The listing builds one solid part. Answer for the finished solid, in the listing's coordinates (mm). Face numbers are marked on the shaded views. Round coordinates to 2 decimals unless told otherwise and drop trailing zeros. Order: outer loops, then holes, each group sorted by start corner. A loop starts at its lowest first (then second) coordinate and runs counter-clockwise, first axis right, second up. Notation, with made-up numbers: M 24,81.25 L 43,81.25 A12 ccw 43,91.25 Z; hole C -30,68.5 d6. An arc over 180 degrees is marked long. Write item = value, one per line. Start each with the question number.
(1) A cutting plane is placed at B-B, the plane x = 230.5. Determine the outline of the cut face in (y, z) (3 decimals).
(2) Each of these flat-tipped pins is pushed along its axis until it touches: pin 1 (1.6 mm diameter, centred on y = 14, z = 23, fed in from -X); pin 2 (2.5 mm diameter, centred on y = 14.5, z = 23.5, fed in from +X). Where does it stop, or does it pass through?
(3) A cutting plane is placed at A-A, the plane y = 14. Determine the outline of the cut face in (x, z) (3 decimals), and give its area (3 significant figures).
(4) A cutting plane is placed at C-C, the plane x = 379.74. Determine the outline of the cut face in (y, z) (3 decimals).
(5) Straight lines are drawn through the part: probe 1 along Y at (x, z) = (350.5, 4.5) (3 decimals); probe 2 along X at (y, z) = (15, 22.5). For each, find the intervals that lie inside material, in ascending order. Write a range as from..to.
(6) For a pull along Y with two mould halves and no side action, classify the marked faces 1, 2 and 3 as released by +Y, released by -Y, zero draft, split by the parting line, or undercut.
from build123d import *

# Parameters (mm, degrees)
SKETCH1_W           = 395.5
SKETCH1_H           = 25.4
SKETCH1_R           = 3.175
BOSS_EXTRUDE1_DEPTH = 25.4
CUT_EXTRUDE1_REACH  = 399.128
SKETCH2_W           = 19.05
SKETCH2_H           = 19.05
SKETCH4_W           = 25.4
SKETCH4_H           = 19.05
CUT_EXTRUDE2_DEPTH  = 38.1
FILLET1_R           = 20


with BuildPart() as part:
    # Sketch1 → Boss-Extrude1 (new body)
    with BuildSketch(Plane(origin=(0, 0, 0), x_dir=(1, 0, 0), z_dir=(0, 1, 0))):
        with Locations((197.75, -12.7)):
            Rectangle(SKETCH1_W, SKETCH1_H)
        with Locations(Location((197.75, -12.7, 0), (0, 0, 270))):
            Circle(SKETCH1_R, mode=Mode.SUBTRACT)
        with Locations(Location((15.76, -12.7, 0), (0, 0, 270))):
            Circle(SKETCH1_R, mode=Mode.SUBTRACT)
        with Locations(Location((379.74, -12.7, 0), (0, 0, 90))):
            Circle(SKETCH1_R, mode=Mode.SUBTRACT)
    extrude(amount=BOSS_EXTRUDE1_DEPTH)

    # Cut-Extrude1: up to this face of the body (flat: up to its plane)
    cut_extrude1_end = Plane(part.part.faces().sort_by_distance((395.5, 12.7, 12.7))[0])
    # Sketch2 → Cut-Extrude1 (cut, up to the picked face)
    with BuildSketch(Plane.ZY, mode=Mode.PRIVATE) as cut_extrude1_sk1:
        with Locations((12.7, 12.7)):
            Rectangle(SKETCH2_W, SKETCH2_H)
    cut_extrude1_tool1 = split(extrude(cut_extrude1_sk1.sketch, amount=-CUT_EXTRUDE1_REACH, mode=Mode.PRIVATE), bisect_by=cut_extrude1_end, keep=Keep.BOTH, mode=Mode.PRIVATE)
    add(cut_extrude1_tool1.solids().sort_by(Axis((0, 12.7, 12.7), (1, 0, 0)))[0], mode=Mode.SUBTRACT)

    # Sketch4 → Cut-Extrude2 (cut)
    with BuildSketch(Plane.ZY):
        with Locations((12.7, 12.7)):
            Rectangle(SKETCH4_W, SKETCH4_H)
    cut_extrude2 = extrude(amount=-CUT_EXTRUDE2_DEPTH, mode=Mode.SUBTRACT)

    # Mirror1: Cut-Extrude2 across plane
    add(cut_extrude2.mirror(Plane.ZY.offset(-197.75)), mode=Mode.SUBTRACT)

    # Fillet1
    # the kernel refuses this fillet: 20 mm, written as the material it takes off along each edge
    with BuildSketch(Plane(origin=(395.5, -50, 0), x_dir=(-1, 0, 0), z_dir=(0, 1, 0)), Plane(origin=(395.5, -27.775, 0), x_dir=(-1, 0, 0), z_dir=(0, 1, 0)), Plane(origin=(0, -27.775, 25.4), x_dir=(1, 0, 0), z_dir=(0, 1, 0))) as fillet1_piece_1:
        with BuildLine():
            CenterArc((FILLET1_R, FILLET1_R), FILLET1_R, 180, 90)
            Line((0, FILLET1_R), (0, 0))
            Line((0, 0), (FILLET1_R, 0))
        make_face()
    extrude(amount=103.175, mode=Mode.SUBTRACT)
    with BuildSketch(Plane(origin=(395.5, -50, 25.4), x_dir=(-1, 0, 0), z_dir=(0, 1, 0)), Plane(origin=(395.5, -27.775, 25.4), x_dir=(-1, 0, 0), z_dir=(0, 1, 0)), Plane(origin=(0, -50, 25.4), x_dir=(0, 0, -1), z_dir=(0, 1, 0)), Plane(origin=(0, -50, 0), x_dir=(1, 0, 0), z_dir=(0, 1, 0)), Plane(origin=(0, -27.775, 0), x_dir=(1, 0, 0), z_dir=(0, 1, 0))) as fillet1_piece_2:
        with BuildLine():
            CenterArc((FILLET1_R, -FILLET1_R), FILLET1_R, 90, 90)
            Line((0, -FILLET1_R), (0, 0))
            Line((0, 0), (FILLET1_R, 0))
        make_face()
    extrude(amount=103.175, mode=Mode.SUBTRACT)


solid = part.part
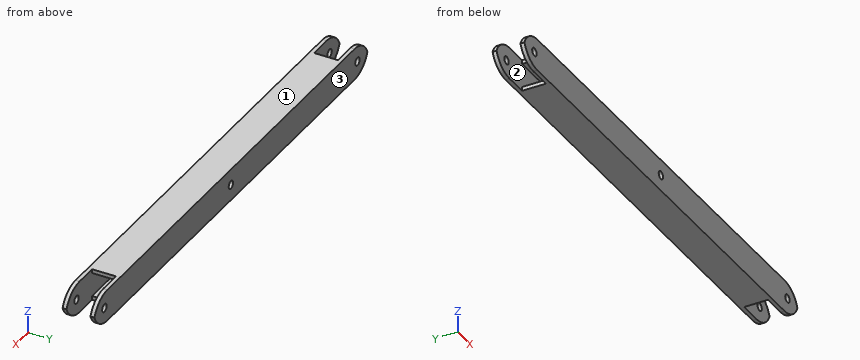
Reported:
q1.outline = M 0,0 L 25.4,0 L 25.4,25.4 L 0,25.4 Z; hole M 3.175,3.175 L 22.225,3.175 L 22.225,22.225 L 3.175,22.225 Z
q2.pin_1 = 38.1
q2.pin_2 = 357.4
q3.outline = M 38.1,0 L 357.4,0 L 357.4,3.175 L 38.1,3.175 Z; M 38.1,22.225 L 357.4,22.225 L 357.4,25.4 L 38.1,25.4 Z
q3.area = 2,030 mm²
q4.outline = M 0,0.455 L 3.175,0.455 L 3.175,9.525 L 0,9.525 Z; M 0,15.875 L 3.175,15.875 L 3.175,24.945 L 0,24.945 Z; M 22.225,0.455 L 25.4,0.455 L 25.4,9.525 L 22.225,9.525 Z; M 22.225,15.875 L 25.4,15.875 L 25.4,24.945 L 22.225,24.945 Z
q5.probe_1 = 0..3.175, 22.225..25.4
q5.probe_2 = 38.1..357.4
q6.face_1 = zero draft
q6.face_2 = undercut
q6.face_3 = released by +Y
